```python
from build123d import *

# Parameters (mm, degrees)
BOSS_EXTRUDE1_DEPTH      = 20
BOSS_EXTRUDE1_DEPTH_BACK = 20
CUT_EXTRUDE1_START       = -10
CUT_EXTRUDE1_DEPTH       = 10
CUT_EXTRUDE3_DEPTH       = 10
FILLET1_R                = 3
FILLET2_R                = 10


with BuildPart() as part:
    # Sketch1 → Boss-Extrude1 (new, two sides: drawn at the far end of the back side and taken through both)
    with BuildSketch(Plane(origin=(0, 0, 0), x_dir=(0, 0, -1), z_dir=(1, 0, 0)).offset(-BOSS_EXTRUDE1_DEPTH_BACK)):
        with BuildLine():
            Line((-50, -20), (50, -20))
            Line((50, -20), (50, 20))
            Line((50, 20), (-50, 20))
            ThreePointArc((-50, 20), (-70, 0), (-50, -20))
        make_face()
    extrude(amount=BOSS_EXTRUDE1_DEPTH + BOSS_EXTRUDE1_DEPTH_BACK)

    # Sketch2 → Cut-Extrude1 (cut)
    with BuildSketch(Plane(origin=(20, 0, 0), x_dir=(0, 0, -1), z_dir=(1, 0, 0)).offset(CUT_EXTRUDE1_START)):
        with BuildLine():
            Line((-2.5, -12.043130914), (40.318290614, 15))
            Line((40.318290614, 15), (-36.771243445, 15))
            ThreePointArc((-36.771243445, 15), (-33.198235095, 10.848995164), (-30.885242753, 5.884390825))
            Line((-30.885242753, 5.884390825), (-2.5, -12.043130914))
        make_face()
        Polygon((45, -15), (45, 12.043130914), (2.181709386, -15), align=None)
        with BuildLine():
            Line((-36.771243445, -15), (-7.181709386, -15))
            Line((-7.181709386, -15), (-30.008501328, -0.583078774))
            ThreePointArc((-30.008501328, -0.583078774), (-31.893143736, -8.493630334), (-36.771243445, -15))
        make_face()
    extrude(amount=CUT_EXTRUDE1_DEPTH, mode=Mode.SUBTRACT)

    # Sketch4 → Cut-Extrude3 (cut)
    with BuildSketch(Plane.ZY.offset(20)):
        with BuildLine():
            Line((2.5, -12.043130914), (30.885242753, 5.884390825))
            ThreePointArc((30.885242753, 5.884390825), (33.198235095, 10.848995164), (36.771243445, 15))
            Line((36.771243445, 15), (-40.318290614, 15))
            Line((-40.318290614, 15), (2.5, -12.043130914))
        make_face()
        with BuildLine():
            Line((7.181709386, -15), (36.771243445, -15))
            ThreePointArc((36.771243445, -15), (31.893143736, -8.493630334), (30.008501328, -0.583078774))
            Line((30.008501328, -0.583078774), (7.181709386, -15))
        make_face()
        Polygon((-45, 12.043130914), (-45, -15), (-2.181709386, -15), align=None)
    extrude(amount=-CUT_EXTRUDE3_DEPTH, mode=Mode.SUBTRACT)

    # Fillet1
    fillet1_edges = [part.edges().sort_by_distance(p)[0] for p in [
        (15, -15, 36.771243445),
        (15, -0.583078774, 30.008501328),
        (15, -15, 7.181709386),
        (15, 12.043130914, -45),
        (15, -15, -45),
        (15, -15, -2.181709386),
        (15, 15, 36.771243445),
        (15, 15, -40.318290614),
        (-15, 15, 36.771243445),
        (-15, 15, -40.318290614),
        (-15, -0.583078774, 30.008501328),
        (-15, -15, 36.771243445),
        (-15, -15, 7.181709386),
        (-15, -15, -2.181709386),
        (-15, -15, -45),
        (-15, 12.043130914, -45),
    ]]
    fillet(fillet1_edges, radius=FILLET1_R)

    # Fillet2
    fillet2_edges = [part.edges().sort_by_distance(p)[0] for p in [
        (15, -12.043130914, 2.5),
        (-15, -12.043130914, 2.5),
    ]]
    fillet(fillet2_edges, radius=FILLET2_R)


solid = part.part
```
Here's how the part is built. I have some questions about the finished solid (model axes, mm). A direction names the side the tool comes from. Coordinates: 2 decimals unless noted, no trailing zeros. Write each loop counter-clockwise with the first axis right and the second up, starting at its lowest first coordinate (ties: lowest second). Pieces come first, ordered by that corner, then holes. Notation, with made-up numbers: (-1, -18) -> (11, -18) arc R28 ccw to (11, 6) -> close; hole circle Ø5 at (88.25, 53.5). An arc over 180 degrees is marked (long way). Use a Markdown table: item, result. Add a question column.
(1) If we section it at C-C, the plane y = 3: Write out the boundary of the cut face in (x, z), and give its area (3 significant figures).
(2) If we section it at B-B, the plane z = 19.5: Write out the boundary of the cut face in (x, y).
(3) If we section it at D-D, the plane x = 0.5: Write out the boundary of the cut face in (y, z).
(4) I'm going to push flat-ended pins straight in: P1, Ø7.5, axis at y = 7.5, z = -0.5, coming from the +X side; P2, Ø7.5, axis at y = -2, z = -31.5, coming from the -X side; P3, Ø5, axis at x = -13.5, y = -7.5, coming from the +Z side. Where does each tip first touch, or does it pass through?
(5) If we section it at A-A, the plane x = 14: Write out the boundary of the cut face in (y, z), and give its area (3 significant figures).
(6) Please list where these lines run through material, in increasing order: line 1 (Z direction, x = 17, y = 0.5); line 2 (Z direction, x = 13.5, y = -8); line 3 (Z direction, x = -15.5, y = -12).
(7) For faces 1 (the cylindrical face through (15.07, -13.51, 32.97)), 2 (the cylindrical face through (-14.93, -2.796, 28.769)), which set-ups out of +Z, -Z, +X, -X, +Y, -Y let a thin tool reach every point of the face, with its end or its side?
(8) We'd pull the mould along Y, two halves only. Please class faces 3 (the flat face through (0, 20, -1)), 4 (the cylindrical face through (14.93, -7.7, 31.54)): +Y half, -Y half, draft (parallel to the pull), parting line (faces both ways), or undercut.
Outcome:
| question | item | result |
|---|---|---|
| 1 | outline | (-20, -50) -> (20, -50) -> (20, -45) -> (10, -45) -> (10, -30.68) -> (20, -30.68) -> (20, -21.32) -> (10, -21.32) -> (10, 26.32) -> (20, 26.32) -> (20, 69.77) -> (-20, 69.77) -> (-20, 26.32) -> (-10, 26.32) -> (-10, -21.32) -> (-20, -21.32) -> (-20, -30.68) -> (-10, -30.68) -> (-10, -45) -> (-20, -45) -> close |
| 1 | area | 3,550 mm^2 |
| 2 | outline | (-20, -20) -> (20, -20) -> (20, -15) -> (10, -15) -> (10, -7.22) -> (20, -7.22) -> (20, -1.31) -> (10, -1.31) -> (10, 15) -> (20, 15) -> (20, 20) -> (-20, 20) -> (-20, 15) -> (-10, 15) -> (-10, -1.31) -> (-20, -1.31) -> (-20, -7.22) -> (-10, -7.22) -> (-10, -15) -> (-20, -15) -> close |
| 3 | outline | (-20, -50) -> (20, -50) -> (20, 50) arc R20 ccw to (-20, 50) -> close |
| 4 | P1 | stops at x = 10 |
| 4 | P2 | stops at x = -10 |
| 4 | P3 | stops at z = 69.36 |
| 5 | outline | (-20, -50) -> (20, -50) -> (20, 50) arc R20 ccw to (-20, 50) -> close; hole (-15, -42) arc R3 ccw to (-12, -45) -> (6.6, -45) arc R3 ccw to (9.14, -40.4) -> (-9.46, -10.95) arc R3 ccw to (-15, -12.55) -> close; hole (-15, 17.55) arc R3 ccw to (-9.46, 15.95) -> (-3.06, 26.09) arc R3 ccw to (-4.87, 30.6) arc R20 cw to (-10.43, 32.94) arc R3 ccw to (-15, 30.38) -> close; hole (-8.67, -2.84) -> (9.46, -31.55) arc R3 ccw to (15, -29.95) -> (15, 30.38) arc R3 ccw to (10.43, 32.94) arc R20 cw to (5.88, 30.89) -> (-8.67, 7.84) arc R10 ccw to start |
| 5 | area | 2,830 mm^2 |
| 6 | line 1 | z = -50 to -45, -26.72 to -17.36, 22.36 to 69.99 |
| 6 | line 2 | z = -50 to -45, -13.27 to -3.9, 8.9 to 18.27, 31.67 to 68.33 |
| 6 | line 3 | z = -50 to -45, -9.55 to 14.55, 33.38 to 66 |
| 7 | face 1 | +X |
| 7 | face 2 | -X |
| 8 | face 3 | +Y half |
| 8 | face 4 | undercut |
